Here's the drawing with two shaded views (mm, measured from the low corner). I have some questions. A direction names the side the tool comes from. Give positions to 0.01 mm unless a question says otherwise; leave off trailing zeros. Loops run counter-clockwise (first coordinate to the right, second up) from the corner with the lowest first, then second, coordinate; pieces in that order, holes last. Notation, with made-up numbers: M 60.25,15 L 80.25,15 A11 cw 80.25,27 Z; hole C 9,13 d9. An arc over 180 degrees is marked long. Use a Markdown table: item, result. Add a question column.
1) Suppose I cut it at A-A on y = 4. List the corners of the cut face in (x, z) for me, and give its area (3 significant figures).
2) Suppose I cut it at D-D on x = 5. List the corners of the cut face in (y, z) for me, and give its area (3 significant figures).
3) Which directions (+Z, -Z, +X, -X, +Y, -Y) give clear straight access to the entire face, cutting with the end or side of a thin tool? Please do the marked faces 4, 5 and 6.
4) We'd pull the mould along Y, two halves only. Please class the marked faces 1, 2 and 3: +Y half, -Y half, draft (parallel to the pull), parting line (faces both ways), or undercut.
5) Will this pin go through, and if not, where does the flat tip stop? pin 1 Ø5 at (x, y) = (8, 4) entering from -Z.
6) Suppose I cut it at C-C on z = 2.9. List the corners of the cut face in (x, y) for me.
7) If I drill on line 1 along X through (y, z) = (3.5, 0.9); line 2 along Y through (x, z) = (5, 1.85), over which ranges is the centre line in solid material (lowest first)? Write a range as [from, to].
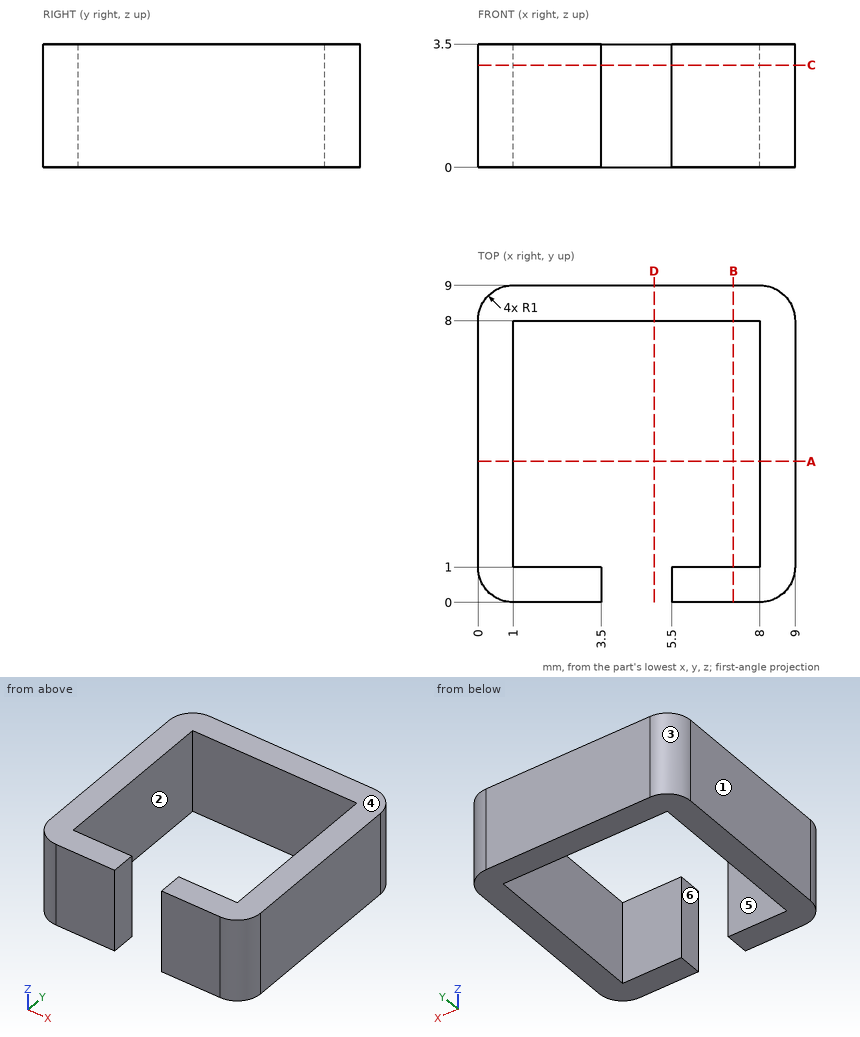
Answer block:
| question | item | result |
|---|---|---|
| 1 | outline | M 0,0 L 1,0 L 1,3.5 L 0,3.5 Z; M 8,0 L 9,0 L 9,3.5 L 8,3.5 Z |
| 1 | area | 7.00 mm^2 |
| 2 | outline | M 8,0 L 9,0 L 9,3.5 L 8,3.5 Z |
| 2 | area | 3.50 mm^2 |
| 3 | face 4 | +Z, +X, -X, +Y, -Y |
| 3 | face 5 | +Z, -Z |
| 3 | face 6 | +Z, -Z, -Y |
| 4 | face 1 | draft |
| 4 | face 2 | undercut |
| 4 | face 3 | +Y half |
| 5 | pin 1 | stops at z = 0 |
| 6 | outline | M 0,1 A1 ccw 1,0 L 3.5,0 L 3.5,1 L 1,1 L 1,8 L 8,8 L 8,1 L 5.5,1 L 5.5,0 L 8,0 A1 ccw 9,1 L 9,8 A1 ccw 8,9 L 1,9 A1 ccw 0,8 Z |
| 7 | line 1 | x = [0, 1], [8, 9] |
| 7 | line 2 | y = [8, 9] |
